Design review of the part built by this model. Coordinates are the model's own, in mm. Face numbers are marked on the shaded views. A direction names the side the tool comes from. Give positions to 0.01 mm unless a question says otherwise; leave off trailing zeros. Loops run counter-clockwise (first coordinate to the right, second up) from the corner with the lowest first, then second, coordinate; pieces in that order, holes last. Notation, with made-up numbers: (24, 71.25) - (56, 71.25) arc R18 cw to (56, 79.25) - close; hole circle Ø9 at (-39.75, 80.25). An arc over 180 degrees is marked (long way). Write each question's results on one line, items separated by ' | '.
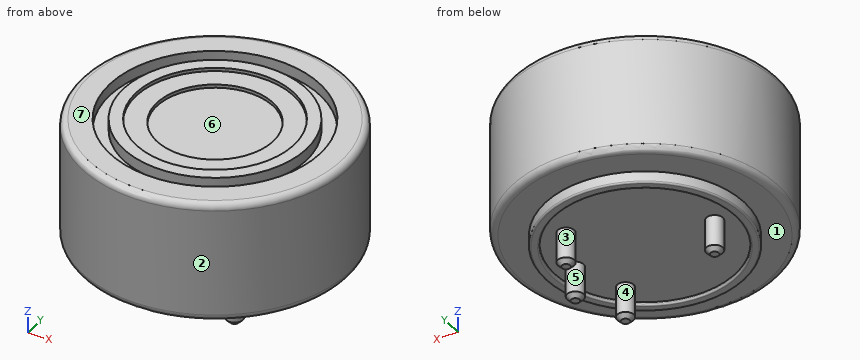
```python
from build123d import *

# Parameters (mm, degrees)
SKETCH_1_R          = 16
EXTRUDE_1_DEPTH     = 14.5
SKETCH_2_R          = 12
SKETCH_2_R_2        = 10.9
EXTRUDE_2_DEPTH     = 1.4
SKETCH_3_R          = 10.9
EXTRUDE_3_DEPTH     = 1
SKETCH_4_R          = 12.65
SKETCH_4_R_2        = 11
CUT_EXTRUDE_1_DEPTH = 1.4
SKETCH_5_R          = 9.5
CUT_EXTRUDE_2_DEPTH = 0.4
SKETCH_6_R          = 7
CUT_EXTRUDE_3_DEPTH = 0.4
SKETCH_7_R          = 1
EXTRUDE_4_DEPTH     = 4.2
CHAMFER_1_SIZE      = 0.5
FILLET_1_R          = 0.8
FILLET_2_R          = 0.2


with BuildPart() as part:
    # Эскиз1 → Бобышка-Вытянуть1 (new body)
    with BuildSketch(Plane.XY):
        with Locations(Location((0, 0, 0), (0, 0, 180))):
            Circle(SKETCH_1_R)
    extrude(amount=EXTRUDE_1_DEPTH)

    # Эскиз2 → Бобышка-Вытянуть2 (add)
    with BuildSketch(Plane(origin=(0, 0, 0), x_dir=(-1, 0, 0), z_dir=(0, 0, -1))):
        with Locations(Location((0, 0, 0), (0, 0, 180))):
            Circle(SKETCH_2_R)
        Circle(SKETCH_2_R_2, mode=Mode.SUBTRACT)
    extrude(amount=EXTRUDE_2_DEPTH)

    # Эскиз3 → Бобышка-Вытянуть3 (add)
    with BuildSketch(Plane(origin=(0, 0, 0), x_dir=(-1, 0, 0), z_dir=(0, 0, -1))):
        Circle(SKETCH_3_R)
    extrude(amount=EXTRUDE_3_DEPTH)

    # Эскиз4 → Вырез-Вытянуть1 (cut)
    with BuildSketch(Plane.XY.offset(14.5)):
        Circle(SKETCH_4_R)
        Circle(SKETCH_4_R_2, mode=Mode.SUBTRACT)
    extrude(amount=-CUT_EXTRUDE_1_DEPTH, mode=Mode.SUBTRACT)

    # Эскиз5 → Вырез-Вытянуть2 (cut)
    with BuildSketch(Plane.XY.offset(14.5)):
        Circle(SKETCH_5_R)
    extrude(amount=-CUT_EXTRUDE_2_DEPTH, mode=Mode.SUBTRACT)

    # Эскиз6 → Вырез-Вытянуть3 (cut)
    with BuildSketch(Plane.XY.offset(14.1)):
        Circle(SKETCH_6_R)
    extrude(amount=-CUT_EXTRUDE_3_DEPTH, mode=Mode.SUBTRACT)

    # Эскиз7 → Бобышка-Вытянуть4 (add)
    with BuildSketch(Plane(origin=(0, 0, -1), x_dir=(-1, 0, 0), z_dir=(0, 0, -1))):
        with Locations((-8.4, 0)):
            Circle(SKETCH_7_R)
        with Locations((8.4, 0)):
            Circle(SKETCH_7_R)
        with Locations((-5.938994048, -5.940399793)):
            Circle(SKETCH_7_R)
        with Locations((-5.938994048, 5.940399793)):
            Circle(SKETCH_7_R)
    extrude(amount=EXTRUDE_4_DEPTH)

    # Фаска1
    chamfer_1_edges = [part.edges().sort_by_distance(p)[0] for p in [
        (9.4, 0, -5.2),
        (-7.4, 0, -5.2),
        (6.938994048, -5.940399793, -5.2),
        (6.938994048, 5.940399793, -5.2),
    ]]
    chamfer(chamfer_1_edges, length=CHAMFER_1_SIZE)

    # Скругление1
    fillet_1_edges = [part.edges().sort_by_distance(p)[0] for p in [
        (16, 0, 0),
        (16, 0, 14.5),
    ]]
    fillet(fillet_1_edges, radius=FILLET_1_R)

    # Скругление2
    fillet_2_edges = [part.edges().sort_by_distance(p)[0] for p in [
        (-12, 0, -1.4),
        (10.9, 0, -1.4),
    ]]
    fillet(fillet_2_edges, radius=FILLET_2_R)


solid = part.part
```
Item 1: Clearance check with flat-ended pins moving along their axes: P1, Ø17, axis at x = 0, y = 0, coming from the +Z side; P2, Ø8, axis at y = 8, z = 2, coming from the -X side; P3, Ø5.5, axis at x = 4, y = -1, coming from the +Z side. State where each tip first meets the part, or that it passes through.
Output values:
P1: stops at z = 14.1 | P2: stops at x = -15.49 | P3: stops at z = 13.7
Item 2: We need section A-A on z = 10.75. Give the boundary of the cut face in (x, y), then the cut area to 3 significant figures.
Output values:
outline: circle Ø32 at (0, 0) | area: 804 mm²
Item 3: Wall thickness on probe 1 along Y at (x, z) = (0, -1.05); probe 2 along Y at (x, z) = (-5, 13.25); probe 3 along Y at (x, z) = (0, 14.25): over which ranges is each line inside the solid? List them lowest first.
Output values:
probe 1: y = -12 to -10.9, 10.9 to 12 | probe 2: y = -15.2 to -11.62, -9.8 to 9.8, 11.62 to 15.2 | probe 3: y = -15.78 to -12.65, -11 to -9.5, 9.5 to 11, 12.65 to 15.78
Item 4: Draft analysis for pull direction Y (two halves, no side actions). For the marked faces 1, 2, 3 and 4, state which applies: +Y half, -Y half, draft (parallel to the pull), parting line (faces both ways), or undercut.
Output values:
face 1: draft | face 2: parting line | face 3: undercut | face 4: undercut
Item 5: We need section B-B on z = -2. Give the boundary of the cut face in (x, y).
Output values:
outline: circle Ø2 at (-8.4, 0); circle Ø2 at (5.94, -5.94); circle Ø2 at (5.94, 5.94); circle Ø2 at (8.4, 0)
Item 6: Tool access review of the marked faces 5, 6 and 7: name each direction out of +Z, -Z, +X, -X, +Y, -Y from which nothing blocks a thin tool from reaching the whole face with its end or side.
Output values:
face 5: -Z | face 6: +Z | face 7: +Z, +X, -X, +Y, -Y
